```python
from build123d import *

# Parameters (mm, degrees)
SKETCH1_W           = 2.7
SKETCH1_H           = 20
BOSS_EXTRUDE1_DEPTH = 20
SKETCH4_RX          = 13
SKETCH4_RY          = 10.172604586
BOSS_EXTRUDE2_DEPTH = 20
REVOLVE1_ANGLE      = 180
CUT_EXTRUDE1_REACH  = 58.934
SKETCH6_R           = 1.64
SKETCH6_W           = 14
SKETCH6_H           = 10
FILLET1_R           = 2
CUT_REVOLVE5_ANGLE  = 180
SKETCH11_R          = 0.86
SKETCH11_R_2        = 1.125
CUT_EXTRUDE5_DEPTH  = 29.98707334


with BuildPart() as part:
    # Sketch1 → Boss-Extrude1 (new body)
    with BuildSketch(Plane(origin=(0, 0, 0), x_dir=(1, 0, 0), z_dir=(0, 1, 0))):
        with Locations((5.15, 10)):
            Rectangle(SKETCH1_W, SKETCH1_H)
    extrude(amount=BOSS_EXTRUDE1_DEPTH)

    # Sketch4 → Boss-Extrude2 (add)
    with BuildSketch(Plane(origin=(0, 20, 0), x_dir=(1, 0, 0), z_dir=(0, 1, 0))):
        with Locations(Location((0, 10), (0, 0, 90))):
            Ellipse(SKETCH4_RX, SKETCH4_RY)
    extrude(amount=BOSS_EXTRUDE2_DEPTH)

    # Sketch5 → Revolve1 (revolve)
    with BuildSketch(Plane(origin=(0, 40, 0), x_dir=(1, 0, 0), z_dir=(0, 1, 0))):
        with BuildLine():
            Line((0, 23), (0, -3))
            add(Edge.make_bspline(
                [(0, -3), (10.172604586, -3.000000114), (10.172604586, 9.999999968), (10.172604586, 23.00000005), (0, 23)],
                knots=[6.283185294, 6.283185294, 6.283185294, 7.853981628, 7.853981628, 9.424777961, 9.424777961, 9.424777961], degree=2, weights=[1, 0.707106779, 1, 0.707106779, 1]))
        make_face()
    revolve(axis=Axis((0, 40, -23), (0, 0, 1)), revolution_arc=REVOLVE1_ANGLE)

    # Sketch6 → Cut-Extrude1 (cut, up to next)
    with BuildSketch(Plane.ZY.offset(-3.8), mode=Mode.PRIVATE) as cut_extrude1_sk1:
        with Locations((-10, 4)):
            Circle(SKETCH6_R)
    cut_extrude1_tool1 = extrude(cut_extrude1_sk1.sketch, amount=-CUT_EXTRUDE1_REACH, mode=Mode.PRIVATE) & part.part
    # Sketch6 → Cut-Extrude1 (cut, up to next)
    with BuildSketch(Plane.ZY.offset(-3.8), mode=Mode.PRIVATE) as cut_extrude1_sk2:
        with Locations((-10, 15)):
            Rectangle(SKETCH6_W, SKETCH6_H)
    cut_extrude1_tool2 = extrude(cut_extrude1_sk2.sketch, amount=-CUT_EXTRUDE1_REACH, mode=Mode.PRIVATE) & part.part
    add(cut_extrude1_tool1.solids().sort_by_distance((3.8, 4, -10))[0], mode=Mode.SUBTRACT)
    add(cut_extrude1_tool2.solids().sort_by_distance((3.8, 15, -10))[0], mode=Mode.SUBTRACT)

    # Fillet1
    fillet1_edges = [part.edges().sort_by_distance(p)[0] for p in [
        (5.15, 10, -17),
        (5.15, 10, -3),
        (5.15, 0, -20),
        (5.15, 0, 0),
    ]]
    fillet(fillet1_edges, radius=FILLET1_R)

    # Sketch10 → Cut-Revolve5 (revolve, cut)
    with BuildSketch(Plane.XZ.offset(-20)):
        with BuildLine():
            Line((0, 0), (0, -20))
            add(Edge.make_bspline(
                [(0, -20), (5.321064319, -20), (5.321064319, -10), (5.321064319, 0), (0, 0)],
                knots=[0, 0, 0, 1.570796327, 1.570796327, 3.141592654, 3.141592654, 3.141592654], degree=2, weights=[1, 0.707106781, 1, 0.707106781, 1]))
        make_face()
    revolve(axis=Axis((0, 20, 0), (0, 0, 1)), revolution_arc=CUT_REVOLVE5_ANGLE, mode=Mode.SUBTRACT)

    # Sketch11 → Cut-Extrude5 (cut)
    with BuildSketch(Plane(origin=(0, 20, 0), x_dir=(-1, 0, 0), z_dir=(0, -1, 0))):
        with Locations(Location((-2.13, 14.83, 0), (0, 0, 90))):
            Circle(SKETCH11_R)
        with Locations(Location((-2.5, 20, 0), (0, 0, 90))):
            Circle(SKETCH11_R_2)
        with Locations(Location((2.5, 20, 0), (0, 0, 90))):
            Circle(SKETCH11_R_2)
        with Locations(Location((-2.5, 0, 0), (0, 0, 90))):
            Circle(SKETCH11_R_2)
        with Locations(Location((2.5, 0, 0), (0, 0, 90))):
            Circle(SKETCH11_R_2)
    extrude(amount=-CUT_EXTRUDE5_DEPTH, mode=Mode.SUBTRACT)


solid = part.part
```
Geometry check sheet. Reference: the model listing, model coordinates, mm. A direction names the side the tool comes from. Give positions to 0.01 mm unless a question says otherwise; leave off trailing zeros. Write each loop counter-clockwise with the first axis right and the second up, starting at its lowest first coordinate (ties: lowest second). Pieces come first, ordered by that corner, then holes. Notation, with made-up numbers: (53.5, -5) - (58.5, -5) arc R22 ccw to (58.5, 9) - close; hole circle Ø10 at (0.25, 2). An arc over 180 degrees is marked (long way). Use a Markdown table: item, result.
Q1. Section check B-B, the plane z = -10. Give the number of separate pieces and of enclosed holes in the cut face, then the cut area to 3 significant figures.
Computed:
| item | result |
|---|---|
| separate pieces | 3 |
| enclosed holes | 0 |
| area | 543 mm² |
Q2. Section check A-A, the plane y = 4. Enter the section's corners in (x, z), then the cut area to 3 significant figures.
Computed:
| item | result |
|---|---|
| outline | (3.8, -20) - (6.5, -20) - (6.5, -11.64) - (3.8, -11.64) - close; (3.8, -8.36) - (6.5, -8.36) - (6.5, 0) - (3.8, 0) - close |
| area | 45.1 mm² |
Q3. Go/stop test with flat-tipped pins: P1, Ø1.4, axis at x = 4.5, y = 16.5, coming from the -Z side; P2, Ø5, axis at y = 33.5, z = -11.5, coming from the -X side; P3, Ø3.5, axis at x = -2.5, z = 0, coming from the -Y side; P4, Ø2.5, axis at x = 2.5, z = -20, coming from the +Y side. Record where each tip stops, or that it passes through.
Computed:
| item | result |
|---|---|
| P1 | stops at z = -20 |
| P2 | stops at x = -10.17 |
| P3 | stops at y = 20 |
| P4 | stops at y = 47.18 |
Q4. Draft check along Z on faces 6 (the face through (-2.162, 33.348, -1.073)), 7 (the face through (3.8, 8, -10)), 8 (the face through (5, 11, -20)). Enter one of: pulls with the +Z half, pulls with the -Z half, needs draft (parallel to the pull), parting line crosses it, or undercut.
Computed:
| item | result |
|---|---|
| face 6 | undercut |
| face 7 | needs draft |
| face 8 | pulls with the -Z half |
Q5. Section check C-C, the plane y = 19. Enter the section's corners in (x, z), then the cut area to 3 significant figures.
Computed:
| item | result |
|---|---|
| outline | (3.8, -20) - (6.5, -20) - (6.5, -17) - (3.8, -17) - close; (3.8, -3) - (6.5, -3) - (6.5, 0) - (3.8, 0) - close |
| area | 16.2 mm² |
Q6. Thickness scan on L1, parallel to Z at x = 2.5, y = 30.5 (3 decimals); L2, parallel to X at y = 28.25, z = 0 (3 decimals); L3, parallel to X at y = 24.5, z = 1. Record the ranges inside material, lowest first. Write a range as [from, to].
Computed:
| item | result |
|---|---|
| L1 | z = [-22.601, -21.125], [-18.875, -15.606], [-14.054, -1.125], [1.125, 2.601] |
| L2 | x = [-6.5, -3.625], [-1.375, 1.375], [3.625, 6.5] |
| L3 | x = [-5.42, -3.02], [-1.98, 1.98], [3.02, 5.42] |
Q7. Set-up check for faces 1 (the face through (5, 16, -3)), 2 (the face through (5, 0, -10)), 3 (the face through (5.17, 0.6, -19.43)), 4 (the face through (6.5, 8, -10)), 5 (the face through (5, 11, 0)): record each of +Z, -Z, +X, -X, +Y, -Y from which the full face is reachable in a straight line by a thin tool's end or side.
Computed:
| item | result |
|---|---|
| face 1 | +X, -X |
| face 2 | +Z, -Z, +X, -X, -Y |
| face 3 | -Z, +X, -X, -Y |
| face 4 | +Z, -Z, +X, -Y |
| face 5 | +Z, +X, -X, -Y |
